Build history of the part. All positions in model axes, mm. A direction names the side the tool comes from. Give positions to 0.01 mm unless a question says otherwise; leave off trailing zeros. Order: outer loops, then holes, each group sorted by start corner. A loop starts at its lowest first (then second) coordinate and runs counter-clockwise, first axis right, second up. Notation, with made-up numbers: (-15, -22.75) -> (1, -22.75) arc R21 ccw to (1, 11.25) -> close; hole circle Ø11 at (72.5, 13). An arc over 180 degrees is marked (long way). Use a Markdown table: item, result. Add a question column.
Autodesk Inventor part; units mm, degrees
ref_plane "XZ Plane" through (0, 0, 0) normal (0, 1, 0) x (-1, 0, 0)
ref_plane "XY Plane" through (0, 0, 0) normal (0, 0, 1) x (1, 0, 0)
sketch "Sketch1" plane through (0, 0, 0) normal (0, 1, 0) x (-1, 0, 0)
  line L0 (-15, -14.4762) -> (15, -14.4762)
  line L1 (15, -14.4762) -> (15, 14.4762)
  line L2 (15, 14.4762) -> (-15, 14.4762)
  line L3 (-15, 14.4762) -> (-15, -14.4762)
  line L4 (-15, -14.4762) -> (15, 14.4762) construction
  line L5 (15, -14.4762) -> (-15, 14.4762) construction
  point P0 (0, 0)
  dimension "d0" = 30
extrude "Extrusion1" add sketch "Sketch1" along normal blind 3.175
sketch "Sketch2" plane through (0, 3.175, 0) normal (0, 1, 0) x (1, 0, 0)
  line L0 (-15, 14.4762) -> (-15, -14.4762)
  line L1 (-15, -14.4762) -> (15, -14.4762)
  line L2 (15, -14.4762) -> (15, 14.4762)
  line L3 (15, 14.4762) -> (-15, 14.4762)
  line L4 (-9.525, -14.4762) -> (-9.525, 14.4762)
  line L5 (0, 20.2667) -> (0, -20.2667)
  line L6 (9.525, -14.4762) -> (9.525, 14.4762)
  point P0 (0, 0)
  dimension "d3" = 19.05
extrude "Extrusion2" add sketch "Sketch2" along normal blind 25.4 contours L3 L4 L1 L0 | L3 L2 L1 L6
sketch "Sketch3" plane through (15, 0, 14.4762) normal (1, 0, 0) x (0, 0, -1)
  line L0 (-5.7905, 0) -> (34.7429, 0) construction
  line L1 (14.4762, -5.715) -> (14.4762, 34.29) construction
  point P0 (14.4762, 0)
  point P1 (14.4762, 20)
  dimension "d6" = 20
hole "Hole1" at (15, 20, 0) direction (-1, 0, 0) diameter 8 end through all
properties part number "Rough_1in_U_Bracket"
(1) Band-saw the part on D-D on x = 13. Give the cut face in (y, z) (3 decimals).
(2) Band-saw the part on C-C on y = 20. Give the cut face in (x, z) (3 decimals).
(3) Band-saw the part on A-A on y = 10. Give the cut face in (x, z) (3 decimals).
(4) Mould opens along X. For faces 3 (the face through (-9.525, 15.7, 0.2)), 4 (the face through (-15, 14, 0)), 5 (the face through (12.224, 16.034, 0.521)) say: released by +X, released by -X, zero draft, split by the parting line, or undercut.
(5) Wall check: probe 1 along Z at (x, y) = (-12.9, 20); probe 2 along X at (y, z) = (14.25, -6.5) (3 decimals); probe 3 along Y at (x, z) = (13, 0) (3 decimals). Give the ranges that are in metal, low to high.
(6) Tool access for faces 1 (the face through (0, 3.175, 0)), 2 (the face through (0, 0, 0)): list every direction of +Z, -Z, +X, -X, +Y, -Y with a clear straight run to the whole face (end or side of a thin tool).
(7) Band-saw the part on B-B on z = 0. Give the cut face in (x, y) (3 decimals).
(8) Pin check, flat tip, straight feed: pin 1 Ø5 at (x, z) = (-1.5, 10) entering from +Y (3 decimals). Stop position of the tip, or through.
Response:
| question | item | result |
|---|---|---|
| 1 | outline | (0, -14.476) -> (28.575, -14.476) -> (28.575, 14.476) -> (0, 14.476) -> close; hole circle Ø8 at (20, 0) |
| 2 | outline | (-15, -14.476) -> (-9.525, -14.476) -> (-9.525, -4) -> (-15, -4) -> close; (-15, 4) -> (-9.525, 4) -> (-9.525, 14.476) -> (-15, 14.476) -> close; (9.525, -14.476) -> (15, -14.476) -> (15, -4) -> (9.525, -4) -> close; (9.525, 4) -> (15, 4) -> (15, 14.476) -> (9.525, 14.476) -> close |
| 3 | outline | (-15, -14.476) -> (-9.525, -14.476) -> (-9.525, 14.476) -> (-15, 14.476) -> close; (9.525, -14.476) -> (15, -14.476) -> (15, 14.476) -> (9.525, 14.476) -> close |
| 4 | face 3 | undercut |
| 4 | face 4 | released by -X |
| 4 | face 5 | zero draft |
| 5 | probe 1 | z = -14.48 to -4, 4 to 14.48 |
| 5 | probe 2 | x = -15 to -9.525, 9.525 to 15 |
| 5 | probe 3 | y = 0 to 16, 24 to 28.575 |
| 6 | face 1 | +Z, -Z, +Y |
| 6 | face 2 | +Z, -Z, +X, -X, -Y |
| 7 | outline | (-15, 0) -> (15, 0) -> (15, 16) -> (9.525, 16) -> (9.525, 3.175) -> (-9.525, 3.175) -> (-9.525, 16) -> (-15, 16) -> close; (-15, 24) -> (-9.525, 24) -> (-9.525, 28.575) -> (-15, 28.575) -> close; (9.525, 24) -> (15, 24) -> (15, 28.575) -> (9.525, 28.575) -> close |
| 8 | pin 1 | stops at y = 3.175 |
